from build123d import *

# Parameters (mm, degrees)
PAD004_DEPTH    = 14
POCKET002_DEPTH = 4.5
SKETCH007_R     = 2.25
HOLE002_DEPTH   = 25


with BuildPart() as part:
    # Sketch009 → Pad004 (new body)
    with BuildSketch(Plane.XY):
        Polygon((0, 0), (0, 8), (-4, 8), (-7.9, 4.1), (-7.9, 2.2), (-3.75, 2.2), (-3.75, 0), align=None)
    pad004 = extrude(amount=PAD004_DEPTH)

    # Mirrored002: Pad004 across Sketch009 V_Axis
    add(pad004.mirror(Plane(origin=(0, 0, 0), x_dir=(0, 0, 1), z_dir=(1, 0, 0))))

    # Sketch008 (on DatumPlane) → Pocket002 (cut)
    with BuildSketch(Plane(origin=(0, 8, 0), x_dir=(-1, 0, 0), z_dir=(0, 1, 0))):
        Polygon((0, 2.727608), (3.7, 4.863804), (3.7, 9.136196), (0, 11.272392), (-3.7, 9.136196), (-3.7, 4.863804), align=None)
    extrude(amount=-POCKET002_DEPTH, mode=Mode.SUBTRACT)

    # Sketch007 (on DatumPlane) → Hole002 (cut)
    with BuildSketch(Plane(origin=(0, 8, 0), x_dir=(-1, 0, 0), z_dir=(0, 1, 0))):
        with Locations((0, 7)):
            Circle(SKETCH007_R)
    extrude(amount=-HOLE002_DEPTH, mode=Mode.SUBTRACT)


solid = part.part
The model under review builds one solid part; all positions refer to its coordinate system, in mm. A direction names the side the tool comes from. Give positions to 0.01 mm unless a question says otherwise; leave off trailing zeros. Order: outer loops, then holes, each group sorted by start corner. A loop starts at its lowest first (then second) coordinate and runs counter-clockwise, first axis right, second up. Notation, with made-up numbers: M 22.5,-23 L 77.5,-23 A8 ccw 77.5,-17 Z; hole C -11.5,8.25 d7. An arc over 180 degrees is marked long. Use one line per item in the form item = value. Start each with the question number.
Item 1: We need section D-D on y = 4.75. Give the boundary of the cut face in (x, z).
Item 2: Insertion check: pin 1 Ø2 at (x, z) = (5.5, 4.5) entering from -Y; pin 2 Ø3 at (y, z) = (6.5, 2.5) entering from -X; pin 3 Ø1.8 at (y, z) = (1, 5) entering from -X. Each pin has a flat end and moves straight along its axis. Give the tip position at first contact, or say it passes through.
Item 3: We need section A-A on z = 7. Give the boundary of the cut face in (x, y).
Item 4: The part is to be moulded in two halves that separate along X. For faces 1 (the flat face through (2, 3.5, 5)), 2 (the flat face through (6, 2.2, 7)), 3 (the flat face through (1.82, 5.78, 10.22)), 4 (the flat face through (7.9, 3, 7)), say which applies: pulls with the +X half, pulls with the -X half, needs draft (parallel to the pull), parting line crosses it, or undercut.
Item 5: We need section C-C on z = 11. Give the boundary of the cut face in (x, y), plus the area to 3 significant figures.
Item 6: We need section B-B on y = 6.25. Give the boundary of the cut face in (x, z).
Item 7: To check wall thickness, follow line 1 along Z through (x, y) = (0, 2.85); line 2 along X through (y, z) = (2, 12.75); line 3 along Y through (x, z) = (-2.5, 5.5). State the ranges of each line that lie inside material, in increasing order. Write a range as from..to.
Item 8: For faces 5 (the flat face through (1.876, 5.781, 3.811)), 6 (the flat face through (-6, 2.2, 7)), 7 (the flat face through (3.75, 1, 7)), 8 (the flat face through (2, 0, 5)), list the 3-axis set-ups (+Z, -Z, +X, -X, +Y, -Y) from which the entire face can be reached by the end or side of a thin tool; tool diameter is ignored.
Completed:
q1.outline = M -7.25,0 L 7.25,0 L 7.25,14 L -7.25,14 Z; hole M -3.7,4.86 L 0,2.73 L 3.7,4.86 L 3.7,9.14 L 0,11.27 L -3.7,9.14 Z
q2.pin_1 = 2.2
q2.pin_2 = -7
q2.pin_3 = -3.75
q3.outline = M -7.9,2.2 L -3.75,2.2 L -3.75,0 L -2.25,0 L -2.25,3.5 L -3.7,3.5 L -3.7,8 L -4,8 L -7.9,4.1 Z; M 2.25,0 L 3.75,0 L 3.75,2.2 L 7.9,2.2 L 7.9,4.1 L 4,8 L 3.7,8 L 3.7,3.5 L 2.25,3.5 Z
q4.face_1 = undercut
q4.face_2 = needs draft
q4.face_3 = undercut
q4.face_4 = pulls with the +X half
q5.outline = M -7.9,2.2 L -3.75,2.2 L -3.75,0 L 3.75,0 L 3.75,2.2 L 7.9,2.2 L 7.9,4.1 L 4,8 L 0.47,8 L 0.47,3.5 L -0.47,3.5 L -0.47,8 L -4,8 L -7.9,4.1 Z
q5.area = 88.7 mm²
q6.outline = M -5.75,0 L 5.75,0 L 5.75,14 L -5.75,14 Z; hole M -3.7,4.86 L 0,2.73 L 3.7,4.86 L 3.7,9.14 L 0,11.27 L -3.7,9.14 Z
q7.line_1 = 0..4.75, 9.25..14
q7.line_2 = -3.75..3.75
q7.line_3 = 0..3.5
q8.face_5 = +Y
q8.face_6 = +Z, -Z, -X, -Y
q8.face_7 = +Z, -Z, +X, -Y
q8.face_8 = +Z, -Z, +X, -X, -Y
